Source: CAD feature listing. Evaluate the final solid. Frame: model axes, mm. A direction names the side the tool comes from. Round coordinates to 2 decimals unless told otherwise and drop trailing zeros. Order: outer loops, then holes, each group sorted by start corner. A loop starts at its lowest first (then second) coordinate and runs counter-clockwise, first axis right, second up. Notation, with made-up numbers: (7, -2) -> (49, -2) arc R19 ccw to (49, 10) -> close; hole circle Ø3 at (48.5, 34.25). An arc over 180 degrees is marked (long way). Answer as CSV lines item,"result". Start each with the question number.
(1) Set-up query: faces 4 (the flat face through (7, -8.1, 8)), 5 (the flat face through (50.5, -12.5, 8.1)), 6 (the flat face through (7, -10.1, 11)), 7 (the cylindrical face through (6.9, -11.2, 3.77)). Return all of +Z, -Z, +X, -X, +Y, -Y with unobstructed straight access to the full face (end or side cutting, diameter ignored); none if empty.
(2) Pull-direction query (Y, two-part tool) for faces 1 (the flat face through (7, 8.1, 8)), 2 (the flat face through (0, 0, 1)), 3 (the cylindrical face through (6.9, 11.2, 3.77)); classes: +Y half, -Y half, draft (parallel to the pull), parting line (faces both ways), or undercut.
(3) Contact query for flat-ended pins moving along their axis: P1, Ø1, axis at x = 3.5, y = -9.5, coming from the +Z side; P2, Ø2.5, axis at x = 6, z = 9.5, coming from the +Y side; P3, Ø1.6, axis at x = 44, z = 1, coming from the -Y side; P4, Ø6, axis at y = 1, z = 7, coming from the +X side. Output: stop coordinate, or through.
(4) Section query D-D (y = 6.5). Output: boundary loops of the cut face in (x, z), plus the area to 3 significant figures.
(5) Section query C-C (z = 9.5). Output: boundary loops of the cut face in (x, y).
(6) Section query B-B (x = 12). Output: boundary loops of the cut face in (y, z).
(7) Section query A-A (z = 17.25). Output: boundary loops of the cut face in (x, y), plus the area to 3 significant figures.
(8) Line query: line 1 along Y through (x, z) = (54, 17.25); line 2 along Y through (x, z) = (9.5, 9.25); line 3 along Z through (x, y) = (16, -5.5). Output: solid intervals per line, ascending. Write a range as from..to.
```python
from build123d import *

# Parameters (mm, degrees)
F0_W        = 2
F0_H        = 13
F0_W_2      = 4
F0_H_2      = 2
F1_DEPTH    = 14
F2_DEPTH    = 64.5
F4_DEPTH    = 14
F5_T1_DEPTH = 14
F5_T3_DEPTH = 14


# Not quite as in the source:
# - a fillet or chamfer that OpenCascade refuses, or shapes differently, is made with other operations: its cross-section is extruded or revolved along the edge and cut away or added


with BuildPart() as f1:
    # F0 (on Right) → F1 (new body)
    with BuildSketch(Plane.YZ):
        Polygon((-10.1, 0), (0, 0), (10.1, 0), (10.1, 2), (8.1, 2), (0, 2), (-8.1, 2), (-10.1, 2), align=None)
        with Locations((-9.1, 8.5)):
            Rectangle(F0_W, F0_H)
        with Locations((9.1, 8.5)):
            Rectangle(F0_W, F0_H)
        with Locations((-12.1, 1)):
            Rectangle(F0_W_2, F0_H_2)
        with Locations((12.1, 1)):
            Rectangle(F0_W_2, F0_H_2)
    extrude(amount=F1_DEPTH)

    # F0 (on Right) → F2 (join)
    with BuildSketch(Plane.YZ):
        with Locations((-12.1, 1)):
            Rectangle(F0_W_2, F0_H_2)
        Polygon((-10.1, 0), (0, 0), (10.1, 0), (10.1, 2), (8.1, 2), (0, 2), (-8.1, 2), (-10.1, 2), align=None)
        with Locations((12.1, 1)):
            Rectangle(F0_W_2, F0_H_2)
    extrude(amount=F2_DEPTH)

    # F3 (on face) → F4 (join)
    with BuildSketch(Plane.YZ.offset(64.5)):
        with BuildLine():
            ThreePointArc((15.1106605022, 19.3068031473), (0, 2), (-15.1106605022, 19.3068031473))
            Line((-15.1106605022, 19.3068031473), (-17.1269396219, 19.3068031473))
            ThreePointArc((-17.1269396219, 19.3068031473), (0, 0), (17.1269396219, 19.3068031473))
            Line((17.1269396219, 19.3068031473), (15.1106605022, 19.3068031473))
        make_face()
    extrude(amount=-F4_DEPTH)

    # F5: fillet of radius 5 on 4 edges, made by hand

    # F5_s2 → F5_t1 (join)
    with BuildSketch(Plane.YZ):
        with BuildLine():
            ThreePointArc((-10.1, 6.8989794856), (-11.2270166538, 3.7367018254), (-14.1, 2))
            Line((-14.1, 2), (-10.1, 2))
            Line((-10.1, 2), (-10.1, 6.8989794856))
        make_face()
        with BuildLine():
            ThreePointArc((10.1, 6.8989794856), (11.2270166538, 3.7367018254), (14.1, 2))
            Line((14.1, 2), (10.1, 2))
            Line((10.1, 2), (10.1, 6.8989794856))
        make_face()
    extrude(amount=F5_T1_DEPTH)

    # F5_s4 → F5_t3 (join)
    with BuildSketch(Plane.YZ.offset(50.5)):
        with BuildLine():
            ThreePointArc((-14.2181121589, 7.4823090427), (-13.3404640704, 4.7587904606), (-14.1, 2))
            Line((-14.1, 2), (-8.0622577483, 2))
            ThreePointArc((-8.0622577483, 2), (-11.4724735306, 4.3680416438), (-14.2181121589, 7.4823090427))
        make_face()
        with BuildLine():
            ThreePointArc((14.2181121589, 7.4823090427), (13.3404640704, 4.7587904606), (14.1, 2))
            Line((14.1, 2), (8.0622577483, 2))
            ThreePointArc((8.0622577483, 2), (11.4724735306, 4.3680416438), (14.2181121589, 7.4823090427))
        make_face()
    extrude(amount=F5_T3_DEPTH)


solid = f1.part
```
Answer block:
1,face 4,"+Z, -X"
1,face 5,"+Z, +Y, -Y"
1,face 6,"+Z, +X, -X, -Y"
1,face 7,"+Z, -X, -Y"
2,face 1,"undercut"
2,face 2,"draft"
2,face 3,"+Y half"
3,P1,"z = 15"
3,P2,"y = 10.1"
3,P3,"y = -14.1"
3,P4,"through"
4,outline,"(0, 0) -> (64.5, 0) -> (64.5, 3.45) -> (50.5, 3.45) -> (50.5, 2) -> (0, 2) -> close"
4,area,"149 mm2"
5,outline,"(0, -10.1) -> (14, -10.1) -> (14, -8.1) -> (0, -8.1) -> close; (0, 8.1) -> (14, 8.1) -> (14, 10.1) -> (0, 10.1) -> close; (50.5, -15.41) -> (64.5, -15.41) -> (64.5, -13.13) -> (50.5, -13.13) -> close; (50.5, 13.13) -> (64.5, 13.13) -> (64.5, 15.41) -> (50.5, 15.41) -> close"
6,outline,"(-14.1, 0) -> (14.1, 0) -> (14.1, 2) arc R5 cw to (10.1, 6.9) -> (10.1, 15) -> (8.1, 15) -> (8.1, 2) -> (-8.1, 2) -> (-8.1, 15) -> (-10.1, 15) -> (-10.1, 6.9) arc R5 cw to (-14.1, 2) -> close"
7,outline,"(50.5, -17.25) -> (64.5, -17.25) -> (64.5, -15.25) -> (50.5, -15.25) -> close; (50.5, 15.25) -> (64.5, 15.25) -> (64.5, 17.25) -> (50.5, 17.25) -> close"
7,area,"56.0 mm2"
8,line 1,"-17.25..-15.25, 15.25..17.25"
8,line 2,"-10.1..-8.1, 8.1..10.1"
8,line 3,"0..2"
